```python
from build123d import *

# Parameters (mm, degrees)
SKETCH_1_R               = 3.25
EXTRUDE_1_DEPTH          = 20
CUT_EXTRUDE_1_DEPTH      = 81.408360659
CUT_EXTRUDE_1_DEPTH_BACK = 81.408360659


with BuildPart() as part:
    # 草圖1 → 填料-伸長1 (new body)
    with BuildSketch(Plane.XY):
        with BuildLine():
            Line((-41, -60), (-40, -60))
            add(Edge.make_bspline(
                [(-44, -6), (-55, -25), (-40, -60)],
                knots=[0, 0, 0, 1, 1, 1], degree=2))
            add(Edge.make_bspline(
                [(-6.5, 2), (-31.607950909, 0.274777248), (-44, -6)],
                knots=[0, 0, 0, 1, 1, 1], degree=2))
            add(Edge.make_bspline(
                [(-6.5, 2), (0, -13), (6.5, 2)],
                knots=[0, 0, 0, 1, 1, 1], degree=2))
            add(Edge.make_bspline(
                [(6.5, 2), (32.228671013, 0.274777248), (44, -6)],
                knots=[0, 0, 0, 1, 1, 1], degree=2))
            add(Edge.make_bspline(
                [(44, -6), (55, -25), (40, -60)],
                knots=[0, 0, 0, 1, 1, 1], degree=2))
            Line((40, -60), (41, -60))
            add(Edge.make_bspline(
                [(45, -3.5), (56, -25), (41, -60)],
                knots=[0, 0, 0, 1, 1, 1], degree=2))
            add(Edge.make_bspline(
                [(-45, -3.5), (0, 12), (45, -3.5)],
                knots=[0, 0, 0, 1, 1, 1], degree=2))
            add(Edge.make_bspline(
                [(-45, -3.5), (-56, -25), (-41, -60)],
                knots=[0, 0, 0, 1, 1, 1], degree=2))
        make_face()
        Circle(SKETCH_1_R, mode=Mode.SUBTRACT)
    extrude(amount=EXTRUDE_1_DEPTH)

    # 草圖2 → 除料-伸長1 (cut, two sides: drawn at the far end of the back side and taken through both)
    with BuildSketch(Plane(origin=(0, 0, 0), x_dir=(0, 0, -1), z_dir=(1, 0, 0)).offset(-CUT_EXTRUDE_1_DEPTH_BACK)):
        Polygon((-24.134552524, -51.791662607), (-16.07391568, -56.330917091), (-3.22546812, -53.625137827), (5.975024699, -51.687588362), (8.544692021, -68.58770729), (2.04714525, -71.745430098), (-25.301795002, -71.006269551), align=None)
    extrude(amount=CUT_EXTRUDE_1_DEPTH + CUT_EXTRUDE_1_DEPTH_BACK, mode=Mode.SUBTRACT)


solid = part.part
```
Geometry: final body of the model. Coordinates: model frame, mm. Round coordinates to 2 decimals unless told otherwise and drop trailing zeros.
Item 1: Mould query, pull axis X, two halves, no side actions, for faces 1 (the face through (42.433, -55.21, 18.064)), 2 (the face through (-2.579, -1.978, 9.86)). Classes: +X half, -X half, draft (parallel to the pull), parting line (faces both ways), or undercut.
Item 2: Material intervals for L1, parallel to Y at x = 0, z = 12.75; L2, parallel to X at y = -12, z = 5.75; L3, parallel to X at y = -42, z = 10.5, sorted ascending.
Item 3: Pin query (flat end, axial travel): P1, Ø8, axis at x = 26.5, z = 12, coming from the +Y side; P2, Ø4, axis at x = -22, z = 6.5, coming from the +Y side; P3, Ø5, axis at x = -28.5, z = 14.5, coming from the -Y side; P4, Ø8.5, axis at x = 0, y = 0, coming from the +Z side. Return the tip coordinate at first contact, or that it passes through.
Item 4: Section query A-A (y = 0). Give the number of separate pieces and of enclosed holes in the cut face, plus the area to 3 significant figures.
Completed:
1. face 1: draft
1. face 2: undercut
2. L1: y = -5.5 to -3.25, 3.25 to 4.25
2. L2: x = -48.2 to -46.7, 46.7 to 48.2
2. L3: x = -47.23 to -46.27, 46.27 to 47.23
3. P1: stops at y = 2.31
3. P2: stops at y = 2.72
3. P3: stops at y = -1.45
3. P4: stops at z = 20
4. separate pieces: 4
4. enclosed holes: 0
4. area: 462 mm2
